from build123d import *

# Parameters (mm, degrees)
SKETCH_1_R      = 1
SKETCH_1_R_2    = 1.75
SKETCH_1_R_3    = 1.5
SKETCH_1_R_4    = 1.25
EXTRUDE_1_DEPTH = 1


with BuildPart() as part:
    # 草图1 → 凸台-拉伸1 (new body)
    with BuildSketch(Plane.XY):
        with BuildLine():
            ThreePointArc((0.223222552, 2.490014396), (-2.5, 0), (0.223222552, -2.490014396))
            ThreePointArc((0.223222552, -2.490014396), (26.917790455, -1.542011473), (53.559359935, -3.472151542))
            ThreePointArc((53.559359935, -3.472151542), (57.5, 0), (53.559359935, 3.472151542))
            ThreePointArc((53.559359935, 3.472151542), (26.917790455, 1.542011473), (0.223222552, 2.490014396))
        make_face()
        Circle(SKETCH_1_R, mode=Mode.SUBTRACT)
        with Locations((54, 0)):
            Circle(SKETCH_1_R, mode=Mode.SUBTRACT)
        with Locations((49.5, 0)):
            Circle(SKETCH_1_R_2, mode=Mode.SUBTRACT)
        with Locations((45, 0)):
            Circle(SKETCH_1_R_3, mode=Mode.SUBTRACT)
        with Locations((40.5, 0)):
            Circle(SKETCH_1_R_4, mode=Mode.SUBTRACT)
        with Locations((36, 0)):
            Circle(SKETCH_1_R, mode=Mode.SUBTRACT)
    extrude(amount=EXTRUDE_1_DEPTH)


solid = part.part
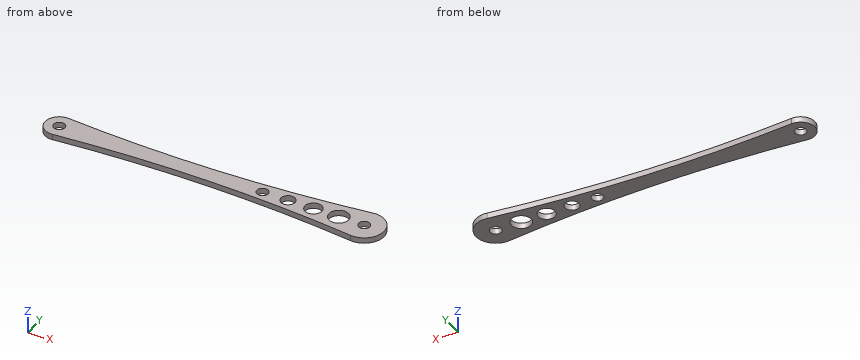
Can you work these out from the model? Positions are in its coordinate system, mm. Give positions to 0.01 mm unless a question says otherwise; leave off trailing zeros. Write each loop counter-clockwise with the first axis right and the second up, starting at its lowest first coordinate (ties: lowest second). Pieces come first, ordered by that corner, then holes. Notation, with made-up numbers: M 70.25,-30 L 107.25,-30 A26 ccw 107.25,-9 Z; hole C -22,2 d7. An arc over 180 degrees is marked long. Answer in a Markdown table with one row per item. Add a question column.
Item 1: Imagine slicing it at C-C, the plane x = 36. Write out the boundary of the cut face in (y, z), plus the area to 3 significant figures.
Item 2: Imagine slicing it at A-A, the plane z = 0.55. Write out the boundary of the cut face in (x, y), plus the area to 3 significant figures.
Item 3: Please list where these lines run through material, in increasing order: L1, parallel to Y at x = 54, z = 0.5; L2, parallel to Y at x = 36, z = 0.7; L3, parallel to Y at x = 29, z = 0.1.
Item 4: For pin 1 Ø3 at (x, y) = (0, 0) entering from +Z, with a flat end and sliding along its axis, tell me the tip position at first contact or that it passes through.
Item 5: Imagine slicing it at B-B, the plane y = 0.5. Write out the boundary of the cut face in (x, z).
Evaluation:
| question | item | result |
|---|---|---|
| 1 | outline | M -1.88,0 L -1,0 L -1,1 L -1.88,1 Z; M 1,0 L 1.88,0 L 1.88,1 L 1,1 Z |
| 1 | area | 1.75 mm² |
| 2 | outline | M 0.22,-2.49 A247.86 cw 53.56,-3.47 A3.5 ccw long 53.56,3.47 A247.86 cw 0.22,2.49 A2.5 ccw long Z; hole C 0,0 d2; hole C 36,0 d2; hole C 40.5,0 d2.5; hole C 45,0 d3; hole C 49.5,0 d3.5; hole C 54,0 d2 |
| 2 | area | 218 mm² |
| 3 | L1 | y = -3.5 to -1, 1 to 3.5 |
| 3 | L2 | y = -1.88 to -1, 1 to 1.88 |
| 3 | L3 | y = -1.59 to 1.59 |
| 4 | pin 1 | stops at z = 1 |
| 5 | outline | M -2.45,0 L -0.87,0 L -0.87,1 L -2.45,1 Z; M 0.87,0 L 35.13,0 L 35.13,1 L 0.87,1 Z; M 36.87,0 L 39.35,0 L 39.35,1 L 36.87,1 Z; M 41.65,0 L 43.59,0 L 43.59,1 L 41.65,1 Z; M 46.41,0 L 47.82,0 L 47.82,1 L 46.41,1 Z; M 51.18,0 L 53.13,0 L 53.13,1 L 51.18,1 Z; M 54.87,0 L 57.46,0 L 57.46,1 L 54.87,1 Z |
